Design review of the part built by this model. Coordinates are the model's own, in mm. A direction names the side the tool comes from. Coordinates: 2 decimals unless noted, no trailing zeros. Loops run counter-clockwise (first coordinate to the right, second up) from the corner with the lowest first, then second, coordinate; pieces in that order, holes last. Notation, with made-up numbers: (58.5, 53.25) - (105.5, 53.25) arc R17 ccw to (105.5, 74.25) - close; hole circle Ø8 at (40, -11.5). An arc over 180 degrees is marked (long way). Return JSON: item names as keys, results as strings. Group by question number.
from build123d import *

# Parameters (mm, degrees)
ESBO_O1_W                = 80
ESBO_O1_H                = 80.95
RESSALTO_EXTRUS_O1_DEPTH = 9.53
ESBO_O2_R                = 2.5
CORTE_EXTRUS_O1_DEPTH    = 20
CORTE_EXTRUS_O2_START    = -20
ESBO_O3_R                = 2.5
CORTE_EXTRUS_O2_DEPTH    = 20


with BuildPart() as part:
    # Esboço1 → Ressalto-extrusão1 (new body)
    with BuildSketch(Plane.XY):
        Rectangle(ESBO_O1_W, ESBO_O1_H)
    extrude(amount=RESSALTO_EXTRUS_O1_DEPTH)

    # Esboço2 → Corte-extrusão1 (cut)
    with BuildSketch(Plane(origin=(0, 40.475, 0), x_dir=(1, 0, 0), z_dir=(0, 1, 0))):
        with Locations(Location((-20, -4.7625, 0), (0, 0, 270))):
            Circle(ESBO_O2_R)
        with Locations(Location((20, -4.7625, 0), (0, 0, 90))):
            Circle(ESBO_O2_R)
    extrude(amount=-CORTE_EXTRUS_O1_DEPTH, mode=Mode.SUBTRACT)

    # Esboço3 → Corte-extrusão2 (cut)
    with BuildSketch(Plane.XZ.offset(40.475).offset(CORTE_EXTRUS_O2_START)):
        with Locations(Location((-20, 4.7625, 0), (0, 0, 90))):
            Circle(ESBO_O3_R)
        with Locations(Location((20, 5, 0), (0, 0, 90))):
            Circle(ESBO_O3_R)
    extrude(amount=CORTE_EXTRUS_O2_DEPTH, mode=Mode.SUBTRACT)


solid = part.part
Item 1: To check wall thickness, follow line 1 (Z direction, x = -20, y = -24.25); line 2 (X direction, y = -32, z = 6); line 3 (Z direction, x = 20, y = -28.25). State the ranges of each line that lie inside material, in increasing order. Write a range as from..to.
Item 2: Add section C-C (z = 5). State the section outline as (x, y) points (3 decimals).
Item 3: Add section A-A (y = 34). State the section outline as (x, z) points, then the cut area to 3 significant figures.
Item 4: Draft analysis for pull direction Z (two halves, no side actions). For faces 4 (the face through (-1, 1, 0)), 5 (the face through (-1, 40.475, 5)), 6 (the face through (20, -20.475, 5)), state which applies: pulls with the +Z half, pulls with the -Z half, needs draft (parallel to the pull), parting line crosses it, or undercut.
Item 5: For faces 1 (the face through (20, 20.475, 5)), 2 (the face through (-1, 1, 9.53)), 3 (the face through (-22.48, -30.34, 4.44)), list the 3-axis set-ups (+Z, -Z, +X, -X, +Y, -Y) from which the entire face can be reached by the end or side of a thin tool; tool diameter is ignored.
Item 6: Add section B-B (x = -20). State the section outline as (y, z) points (1 decimal), then the cut area to 3 significant figures.
Item 7: For P1, Ø4, axis at x = 20, z = 5, coming from the -Y side (3 decimals); P2, Ø1.5, axis at x = -20, z = 5.5, coming from the +Y side (3 decimals), all flat-tipped, find the tip position at first contact; note any pin that passes through.
Answers below:
{
 "1": {"line 1": "z = 0..2.26, 7.26..9.53", "line 2": "x = -40..-22.17, -17.83..17.71, 22.29..40", "line 3": "z = 0..2.5, 7.5..9.53"},
 "2": {"outline": "(-40, -40.475) - (-22.489, -40.475) - (-22.489, -20.475) - (-17.511, -20.475) - (-17.511, -40.475) - (17.5, -40.475) - (17.5, -20.475) - (22.5, -20.475) - (22.5, -40.475) - (40, -40.475) - (40, 40.475) - (22.489, 40.475) - (22.489, 20.475) - (17.511, 20.475) - (17.511, 40.475) - (-17.511, 40.475) - (-17.511, 20.475) - (-22.489, 20.475) - (-22.489, 40.475) - (-40, 40.475) - close"},
 "3": {"outline": "(-40, 0) - (40, 0) - (40, 9.53) - (-40, 9.53) - close; hole circle Ø5 at (-20, 4.76); hole circle Ø5 at (20, 4.76)", "area": "723 mm^2"},
 "4": {"face 4": "pulls with the -Z half", "face 5": "needs draft", "face 6": "undercut"},
 "5": {"face 1": "+Y", "face 2": "+Z, +X, -X, +Y, -Y", "face 3": "-Y"},
 "6": {"outline": "(-40.5, 0) - (40.5, 0) - (40.5, 2.3) - (20.5, 2.3) - (20.5, 7.3) - (40.5, 7.3) - (40.5, 9.5) - (-40.5, 9.5) - (-40.5, 7.3) - (-20.5, 7.3) - (-20.5, 2.3) - (-40.5, 2.3) - close", "area": "571 mm^2"},
 "7": {"P1": "stops at y = -20.475", "P2": "stops at y = 20.475"}
}
